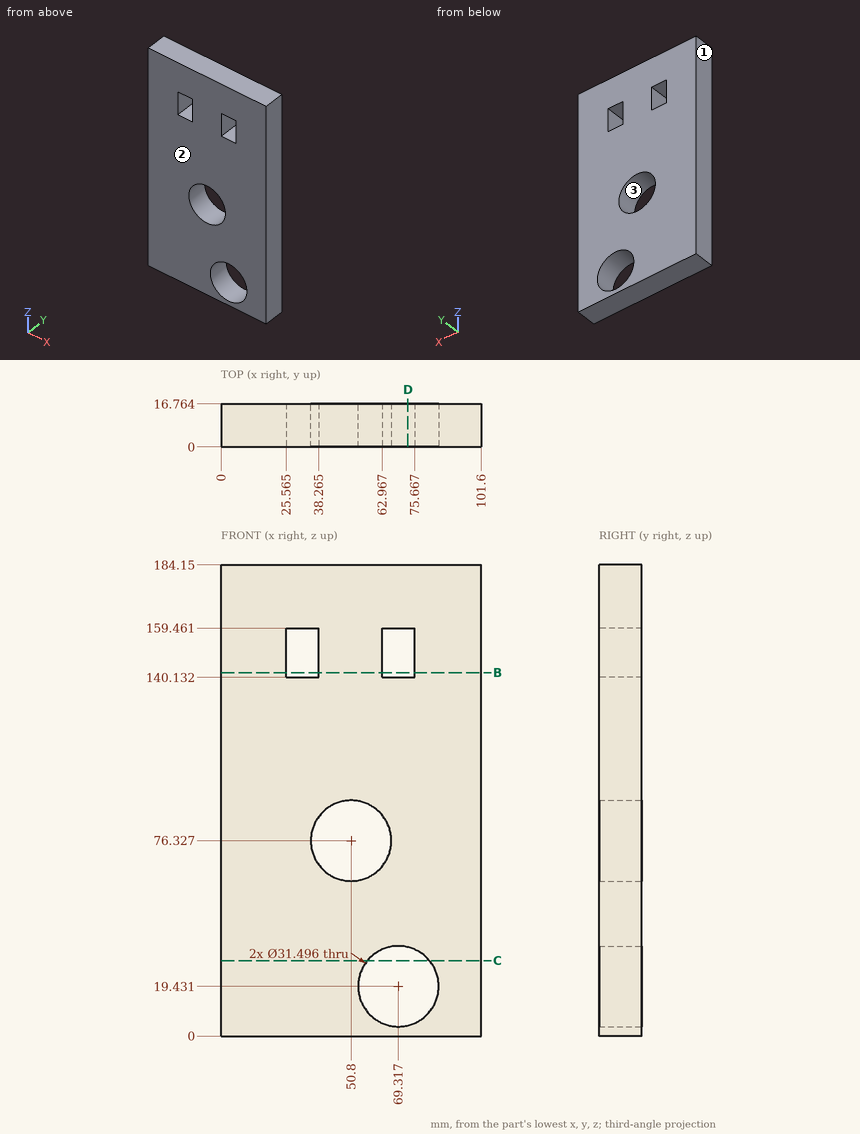
Design review of the part shown in the three views and the two pictorial views. Dimensions are in mm from the part's minimum x, y and z. Round coordinates to 2 decimals unless told otherwise and drop trailing zeros. Loops run counter-clockwise (first coordinate to the right, second up) from the corner with the lowest first, then second, coordinate; pieces in that order, holes last.
(1) We need section D-D (x = 73). Give the boundary of the cut face in (y, z).
Returned:
outline: (0, 0) - (16.76, 0) - (16.76, 4.12) - (0, 4.12) - close; (0, 34.74) - (16.76, 34.74) - (16.76, 140.13) - (0, 140.13) - close; (0, 159.46) - (16.76, 159.46) - (16.76, 184.15) - (0, 184.15) - close
(2) Wall thickness on line 1 along X through (y, z) = (1, 141) (1 decimal); line 2 along X through (y, z) = (4.75, 12); line 3 along X through (y, z) = (5.5, 17) (1 decimal): over which ranges is each line inside the solid? List them lowest first.
Returned:
line 1: x = 0 to 25.6, 38.3 to 63, 75.7 to 101.6
line 2: x = 0 to 55.43, 83.2 to 101.6
line 3: x = 0 to 53.8, 84.9 to 101.6
(3) Clearance check with a flat-ended pin moving along its axis: P1, Ø25, axis at x = 69.32, z = 19.43, coming from the -Y side. State where the tip first meets the part, or that it passes through.
Returned:
P1: passes through
(4) We need section B-B (z = 142). Give the boundary of the cut face in (x, y) (1 decimal).
Returned:
outline: (0, 0) - (25.6, 0) - (25.6, 16.8) - (0, 16.8) - close; (38.3, 0) - (63, 0) - (63, 16.8) - (38.3, 16.8) - close; (75.7, 0) - (101.6, 0) - (101.6, 16.8) - (75.7, 16.8) - close
(5) Mouldability with a two-part tool opening along X and no side actions: class the marked faces 1, 2 and 3 as released by +X, released by -X, zero draft, split by the parting line, or undercut.
Returned:
face 1: released by -X
face 2: zero draft
face 3: undercut
(6) We need section C-C (z = 29.5). Give the boundary of the cut face in (x, y) (1 decimal), plus the area to 3 significant figures.
Returned:
outline: (0, 0) - (57.2, 0) - (57.2, 16.8) - (0, 16.8) - close; (81.4, 0) - (101.6, 0) - (101.6, 16.8) - (81.4, 16.8) - close
area: 1,300 mm2
